Input: part model. Units: mm. Frame: model coordinates. Give positions to 0.01 mm unless a question says otherwise; leave off trailing zeros. Order: outer loops, then holes, each group sorted by start corner. A loop starts at its lowest first (then second) coordinate and runs counter-clockwise, first axis right, second up.
```python
from build123d import *

# Parameters (mm, degrees)
BOSS_EXTRUDE1_DEPTH   = 4
M3_TAPPED_HOLE1_D     = 2.5
M3_TAPPED_HOLE1_DEPTH = 17.5
M3_TAPPED_HOLE1_TIP   = 0.751075774


with BuildPart() as part:
    # Sketch1 → Boss-Extrude1 (new, symmetric)
    with BuildSketch(Plane(origin=(0, 0, 0), x_dir=(1, 0, 0), z_dir=(0, 1, 0))):
        Polygon((2.3, -1.327905619), (2.3, 1.327905619), (0, 2.655811238), (-2.3, 1.327905619), (-2.3, -1.327905619), (0, -2.655811238), align=None)
    extrude(amount=BOSS_EXTRUDE1_DEPTH, both=True)

    # M3 Tapped Hole1
    with Locations(Plane(origin=(0, 4, 0), x_dir=(1, 0, 0), z_dir=(0, 1, 0))):
        with Locations((0, 0)):
            Hole(M3_TAPPED_HOLE1_D / 2, depth=M3_TAPPED_HOLE1_DEPTH)
            with Locations((0, 0, -(M3_TAPPED_HOLE1_DEPTH + M3_TAPPED_HOLE1_TIP / 2))):  # 118° drill point
                Cone(0, M3_TAPPED_HOLE1_D / 2, M3_TAPPED_HOLE1_TIP, mode=Mode.SUBTRACT)


solid = part.part
```
1) Cut plane C-C (x = 0.9). Return the cut outline in (y, z).
2) Line query: probe 1 along X at (y, z) = (0.5, 0.2); probe 2 along Z at (x, y) = (-0.9, 0.5); probe 3 along Z at (x, y) = (1.05, -2). Output: solid intervals per line, ascending.
3) Cut plane B-B (z = 0). Return the cut outline in (x, y).
4) Cut plane A-A (y = -0.5). Return the cut outline in (x, z), then the cut area to 3 significant figures.
5) Cut plane D-D (z = 2.1). Return the cut outline in (x, y), then the cut area to 3 significant figures.
6) First-contact query: P1, Ø1.5, axis at x = 0, z = 0, coming from the -Y side; P2, Ø1, axis at y = 1.5, z = 2, coming from the +X side; P3, Ø1, axis at x = -1.5, y = 1, coming from the +Z side. Flat tips, straight axial feed; report the tip coordinate or a pass-through.
7) Pull-direction query (X, two-part tool) for faces 1 (the face through (0.27, -0.06, 1.22)), 2 (the face through (-1, 4, 1)), 3 (the face through (-2.3, 0, 0)); classes: pulls with the +X half, pulls with the -X half, needs draft (parallel to the pull), parting line crosses it, or undercut.
Geometry says:
1. outline: (-4, -2.14) - (4, -2.14) - (4, -0.87) - (-4, -0.87) - close; (-4, 0.87) - (4, 0.87) - (4, 2.14) - (-4, 2.14) - close
2. probe 1: x = -2.3 to -1.23, 1.23 to 2.3
2. probe 2: z = -2.14 to -0.87, 0.87 to 2.14
2. probe 3: z = -2.05 to -0.68, 0.68 to 2.05
3. outline: (-2.3, -4) - (-1.25, -4) - (-1.25, 4) - (-2.3, 4) - close; (1.25, -4) - (2.3, -4) - (2.3, 4) - (1.25, 4) - close
4. outline: (-2.3, -1.33) - (0, -2.66) - (2.3, -1.33) - (2.3, 1.33) - (0, 2.66) - (-2.3, 1.33) - close; hole circle Ø2.5 at (0, 0)
4. area: 13.4 mm2
5. outline: (-0.96, -4) - (0.96, -4) - (0.96, 4) - (-0.96, 4) - close
5. area: 15.4 mm2
6. P1: passes through
6. P2: stops at x = 2
6. P3: stops at z = 2.08
7. face 1: undercut
7. face 2: needs draft
7. face 3: pulls with the -X half
